from build123d import *

# Parameters (mm, degrees)
F0_W     = 152.209915
F0_H     = 152.209915
F1_DEPTH = 7.62
F3_DEPTH = 7.62
F4_W     = 6.424934
F4_H     = 7.163491
F4_H_2   = 137.427088
F4_W_2   = 139.438458
F4_H_3   = 6.655872
F4_W_3   = 5.60908
F5_DEPTH = 10.16


with BuildPart() as f1:
    # F0 (on Front) → F1 (new body)
    with BuildSketch(Plane.XZ):
        with Locations((-0.173558, 0.173558)):
            Rectangle(F0_W, F0_H)
    extrude(amount=F1_DEPTH)

    # F2 (on Front) → F3 (cut)
    with BuildSketch(Plane.XZ):
        Polygon((60.583096, 2.209843), (76.038271, 40.064868), (76.211937, 76.357067), (17.343326, 76.357067), (3.103723, 62.291671), (26.894279, 59.166025), (6.055835, 43.885101), (52.942332, 55.519439), (41.654844, 8.461132), (57.804637, 27.388643), align=None)
    extrude(amount=F3_DEPTH, mode=Mode.SUBTRACT)

    # F4 (on Front) → F5 (join)
    with BuildSketch(Plane.XZ):
        with Locations((-72.797306, 72.428027)):
            Rectangle(F4_W, F4_H)
        Polygon((9.771794, 76.009773), (-69.584839, 76.009773), (-69.584839, 68.846282), (-69.584839, -68.580806), (69.853619, -68.580806), (75.462699, -68.580806), (75.572275, 38.133189), (60.446158, 1.799743), (57.562228, 26.590804), (41.742637, 7.708041), (40.805306, 7.83694), (52.3897, 54.794144), (5.653567, 43.706257), (25.945945, 59.105508), (2.954097, 62.26727), (16.829018, 76.009773), align=None)
        with Locations((-72.797306, 0.132738)):
            Rectangle(F4_W, F4_H_2)
        Polygon((-69.584839, -68.580806), (-76.009773, -68.580806), (-76.009773, -68.638086), (-76.009773, -75.236678), (-69.584839, -75.236678), align=None)
        with Locations((0.13439, -71.908742)):
            Rectangle(F4_W_2, F4_H_3)
        with Locations((72.658159, -71.908742)):
            Rectangle(F4_W_3, F4_H_3)
    extrude(amount=-F5_DEPTH)


solid = f1.part
Geometry: final body of the model. Coordinates: model frame, mm. A direction names the side the tool comes from. Coordinates: 2 decimals unless noted, no trailing zeros. Loops run counter-clockwise (first coordinate to the right, second up) from the corner with the lowest first, then second, coordinate; pieces in that order, holes last. Notation, with made-up numbers: M -0.5,-24 L 25.5,-24 A20 ccw 25.5,-16 Z; hole C 15.5,29.25 d2. An arc over 180 degrees is marked long. One line per item, written item: value. Start each with the question number.
1) Cut plane B-B (x = 48). Return loops of the section in (y, z).
2) Cut plane C-C (z = 18). Return loops of the section in (x, y), then the cut area to 3 significant figures.
3) Material intervals for L1, parallel to Z at x = 15, y = -5; L2, parallel to Z at x = 12, y = -2; L3, parallel to Z at x = -20.5, y = 7.5, sorted ascending. Write a range as from..to.
4) Cut plane D-D (y = 4.5). Return loops of the section in (x, z), then the cut area to 3 significant figures.
5) Reachability of faces 4 (the flat face through (49.76, 5.01, 17.28)), 5 (the flat face through (10.3, -3.8, 69.4)), 6 (the flat face through (29.17, -3.76, 49.62)) from +Z, -Z, +X, -X, +Y, -Y: full face, straight path, thin tool, end or side. Return the list, or none.
6) Cut plane A-A (y = -4.25). Return loops of the section in (x, z).
7) Draft query along Z for faces 1 (the flat face through (-1, 5, -75.237)), 2 (the flat face through (29.35, 5.01, 49.33)), 3 (the flat face through (-30, -4, 76.279)). Return one class per face: released by +Z, released by -Z, zero draft, split by the parting line, or undercut.
8) Pin query (flat end, axial travel): P1, Ø3.5, axis at y = 4.5, z = -73, coming from the +X side; P2, Ø8, axis at x = -20.5, y = 7.5, coming from the -Z side; P3, Ø5, axis at x = -72, y = 7.5, coming from the +Z side. Return the tip coordinate at first contact, or that it passes through.
Evaluation:
1. outline: M -7.62,-75.93 L 0,-75.93 L 0,-75.24 L 10.16,-75.24 L 10.16,15.18 L 0,15.18 L 0,15.9 L -7.62,15.9 Z; M -7.62,34.91 L 0,34.91 L 0,37 L 10.16,37 L 10.16,53.75 L 0,53.75 L 0,54.29 L -7.62,54.29 Z
2. outline: M -76.28,-7.62 L 43.94,-7.62 L 43.94,0 L 43.31,0 L 43.31,10.16 L -76.01,10.16 L -76.01,0 L -76.28,0 Z; M 49.79,-7.62 L 58.84,-7.62 L 58.84,0 L 58.56,0 L 58.56,10.16 L 50.37,10.16 L 50.37,0 L 49.79,0 Z; M 67.03,-7.62 L 75.93,-7.62 L 75.93,0 L 75.55,0 L 75.55,10.16 L 67.19,10.16 L 67.19,0 L 67.03,0 Z
2. area: 2,430 mm^2
3. L1: -75.93..46.1, 50.44..60.73, 74.04..76.28
3. L2: -75.93..45.36, 48.24..61.12, 71.08..76.28
3. L3: -75.24..76.01
4. outline: M -76.01,-75.24 L 75.46,-75.24 L 75.46,-68.58 L 75.57,38.13 L 60.45,1.8 L 57.56,26.59 L 41.74,7.71 L 40.81,7.84 L 52.39,54.79 L 5.65,43.71 L 25.95,59.11 L 2.95,62.27 L 16.83,76.01 L -76.01,76.01 Z
4. area: 20,400 mm^2
5. face 4: +Y
5. face 5: +X, +Y, -Y
5. face 6: +Y, -Y
6. outline: M -76.28,-75.93 L 75.93,-75.93 L 75.93,39.8 L 60.58,2.21 L 57.8,27.39 L 41.65,8.46 L 52.94,55.52 L 6.06,43.89 L 26.89,59.17 L 3.1,62.29 L 17.26,76.28 L -76.28,76.28 Z
7. face 1: released by -Z
7. face 2: undercut
7. face 3: released by +Z
8. P1: x = 75.46
8. P2: z = -75.24
8. P3: z = 76.01
